```python
from build123d import *

# Parameters (mm, degrees)
F0_W     = 114.3
F0_H     = 50.8
F1_DEPTH = 38.1
F2_SIZE2 = 21.3131306319
F2_SIZE  = 25.4
F3_SIZE  = 12.69999
F4_SIZE2 = 8.098395
F4_SIZE  = 38.09999


# Not quite as in the source:
# - a fillet or chamfer is up to 0.001 mm smaller than in the source, because OpenCascade refuses the exact size


with BuildPart() as f1:
    # F0 (on Top) → F1 (new body)
    with BuildSketch(Plane.XY):
        with Locations((4.716448799, -1.0087825358)):
            Rectangle(F0_W, F0_H)
    extrude(amount=F1_DEPTH)

    # F2
    f2_edges = [f1.edges().sort_by_distance(p)[0] for p in [
        (-52.433551, -1.008783, 0),
    ]]
    f2_side = f1.faces().sort_by_distance((-52.433551, -1.008783, 19.05))[0]
    chamfer(f2_edges, length=F2_SIZE, length2=F2_SIZE2, reference=f2_side)

    # F3 (size 12.7 in the source; OpenCascade refuses exactly that, so slightly less here)
    f3_edges = [f1.edges().sort_by_distance(p)[0] for p in [
        (-52.433551, -1.008783, 38.1),
    ]]
    chamfer(f3_edges, length=F3_SIZE)

    # F4 (size 38.1 and 8.0984049996 in the source; OpenCascade refuses exactly that, so slightly less here)
    f4_edges = [f1.edges().sort_by_distance(p)[0] for p in [
        (61.866449, -1.008783, 38.1),
    ]]
    f4_side = f1.faces().sort_by_distance((61.866449, -1.008783, 19.05))[0]
    chamfer(f4_edges, length=F4_SIZE, length2=F4_SIZE2, reference=f4_side)


solid = f1.part
```
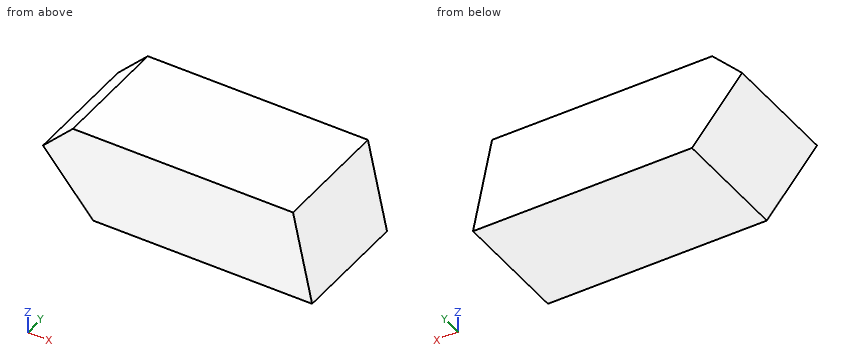
The model under review builds one solid part; all positions refer to its coordinate system, in mm. Give positions to 0.01 mm unless a question says otherwise; leave off trailing zeros. Write each loop counter-clockwise with the first axis right and the second up, starting at its lowest first coordinate (ties: lowest second). Pieces come first, ordered by that corner, then holes. Notation, with made-up numbers: M 70.5,2.25 L 97.5,2.25 A26 cw 97.5,18.25 Z; hole C -31,-28 d6. An arc over 180 degrees is marked long. Write each question's results on one line, items separated by ' | '. Start each with the question number.
1. For probe 1 along X at (y, z) = (-17, 9); probe 2 along X at (y, z) = (9, 16), list the stretches that pass through material, from the lowest coordinate up. Write a range as [from, to].
2. We need section C-C (x = -41). Write out the cut boundary in (y, z), and give its area (3 significant figures).
3. We need section B-B (z = 12.5). Write out the cut boundary in (x, y).
4. Insertion check: pin 1 Ø10 at (x, y) = (43, -0.5) entering from -Z; pin 2 Ø3 at (y, z) = (-7.5, 14) entering from -X. Each pin has a flat end and moves straight along its axis. Give the tip position at first contact, or say it passes through.
Results found:
1) probe 1: x = [-38.67, 59.95] | probe 2: x = [-44.55, 58.47]
2) outline: M -26.41,11.77 L 24.39,11.77 L 24.39,36.83 L -26.41,36.83 Z | area: 1,270 mm^2
3) outline: M -41.61,-26.41 L 59.21,-26.41 L 59.21,24.39 L -41.61,24.39 Z
4) pin 1: stops at z = 0 | pin 2: stops at x = -44.13
